```python
from build123d import *

# Parameters (mm, degrees)
F1_DEPTH = 10
F2_START = 6.1
F2_DEPTH = 3.9


with BuildPart() as f1:
    # F0 (on Front) → F1 (new body)
    with BuildSketch(Plane.XZ):
        with BuildLine():
            Line((-10.0713614853, 99.2132068528), (-89.767584656, 99.2132068528))
            Line((-89.767584656, 99.2132068528), (-204.1870618351, 99.2132068528))
            Line((-204.1870618351, 99.2132068528), (-223.9194730707, 95.7754404094))
            Line((-223.9194730707, 95.7754404094), (-214.9214308969, 56.800637818))
            Line((-214.9214308969, 56.800637818), (-199.3315098604, 60.3998546875))
            ThreePointArc((-199.3315098604, 60.3998546875), (-196.3120285861, 59.8945668129), (-194.5342253839, 57.4021786457))
            Line((-194.5342253839, 57.4021786457), (-182.4993439765, 5.2733801797))
            ThreePointArc((-182.4993439765, 5.2733801797), (-183.004631851, 2.2538989054), (-185.4970200182, 0.4760957032))
            Line((-185.4970200182, 0.4760957032), (-201.0869410548, -3.1231211663))
            Line((-201.0869410548, -3.1231211663), (-179.246252088, -97.7255385038))
            Line((-179.246252088, -97.7255385038), (-49.9194730707, -97.7255385038))
            Line((-49.9194730707, -97.7255385038), (79.4073059466, -97.7255385038))
            Line((79.4073059466, -97.7255385038), (101.2479949134, -3.1231211663))
            Line((101.2479949134, -3.1231211663), (85.6580738768, 0.4760957032))
            ThreePointArc((85.6580738768, 0.4760957032), (83.1656857096, 2.2538989054), (82.6603978351, 5.2733801797))
            Line((82.6603978351, 5.2733801797), (94.6952792425, 57.4021786457))
            ThreePointArc((94.6952792425, 57.4021786457), (96.4730824447, 59.8945668129), (99.492563719, 60.3998546875))
            Line((99.492563719, 60.3998546875), (115.0824847556, 56.800637818))
            Line((115.0824847556, 56.800637818), (124.0805269293, 95.7754404094))
            Line((124.0805269293, 95.7754404094), (104.3481156937, 99.2132068528))
            Line((104.3481156937, 99.2132068528), (-10.0713614853, 99.2132068528))
        make_face()
        with BuildLine():
            Line((-146.7194564495, -12.6849211634), (-142.1879175143, -10.5718298547))
            Line((-142.1879175143, -10.5718298547), (-69.6832945513, 23.2376310846))
            Line((-69.6832945513, 23.2376310846), (-65.1517556162, 25.3507223933))
            ThreePointArc((-65.1517556162, 25.3507223933), (-51.7296025235, 20.4654581878), (-56.614866729, 7.0433050951))
            Line((-56.614866729, 7.0433050951), (-61.1464056642, 4.9302137864))
            Line((-61.1464056642, 4.9302137864), (-133.6510286271, -28.8792471528))
            Line((-133.6510286271, -28.8792471528), (-138.1825675623, -30.9923384615))
            ThreePointArc((-138.1825675623, -30.9923384615), (-151.6047206549, -26.107074256), (-146.7194564495, -12.6849211634))
        make_face(mode=Mode.SUBTRACT)
        with BuildLine():
            Line((38.3436214209, -30.9923384615), (33.8120824857, -28.8792471528))
            Line((33.8120824857, -28.8792471528), (-38.6925404772, 4.9302137864))
            Line((-38.6925404772, 4.9302137864), (-43.2240794124, 7.0433050951))
            ThreePointArc((-43.2240794124, 7.0433050951), (-48.1093436179, 20.4654581878), (-34.6871905252, 25.3507223933))
            Line((-34.6871905252, 25.3507223933), (-30.15565159, 23.2376310846))
            Line((-30.15565159, 23.2376310846), (42.3489713729, -10.5718298547))
            Line((42.3489713729, -10.5718298547), (46.8805103081, -12.6849211634))
            ThreePointArc((46.8805103081, -12.6849211634), (51.7657745136, -26.107074256), (38.3436214209, -30.9923384615))
        make_face(mode=Mode.SUBTRACT)
        with BuildLine():
            ThreePointArc((-115.4963022827, 15.004871972), (-132.7723409168, 21.2928358008), (-126.484377088, 38.5688744349))
            Line((-126.484377088, 38.5688744349), (-117.4212992176, 42.7950570523))
            ThreePointArc((-117.4212992176, 42.7950570523), (-100.1452605835, 36.5070932235), (-106.4332244123, 19.2310545894))
            Line((-106.4332244123, 19.2310545894), (-115.4963022827, 15.004871972))
        make_face(mode=Mode.SUBTRACT)
        with BuildLine():
            Line((-90.729683986, 68.371758879), (-163.234306949, 34.5622979397))
            Line((-163.234306949, 34.5622979397), (-167.7658458841, 32.449206631))
            ThreePointArc((-167.7658458841, 32.449206631), (-181.1879989768, 37.3344708365), (-176.3027347713, 50.7566239292))
            Line((-176.3027347713, 50.7566239292), (-171.7711958361, 52.8697152379))
            Line((-171.7711958361, 52.8697152379), (-99.2665728732, 86.6791761771))
            Line((-99.2665728732, 86.6791761771), (-94.735033938, 88.7922674858))
            ThreePointArc((-94.735033938, 88.7922674858), (-81.3128808454, 83.9070032804), (-86.1981450508, 70.4848501877))
            Line((-86.1981450508, 70.4848501877), (-90.729683986, 68.371758879))
        make_face(mode=Mode.SUBTRACT)
        with BuildLine():
            ThreePointArc((26.6454309466, 38.5688744349), (32.9333947754, 21.2928358008), (15.6573561413, 15.004871972))
            Line((15.6573561413, 15.004871972), (6.594278271, 19.2310545894))
            ThreePointArc((6.594278271, 19.2310545894), (0.3063144421, 36.5070932235), (17.5823530762, 42.7950570523))
            Line((17.5823530762, 42.7950570523), (26.6454309466, 38.5688744349))
        make_face(mode=Mode.SUBTRACT)
        with BuildLine():
            Line((-0.5723732682, 86.6791761771), (71.9322496947, 52.8697152379))
            Line((71.9322496947, 52.8697152379), (76.4637886299, 50.7566239292))
            ThreePointArc((76.4637886299, 50.7566239292), (81.3490528354, 37.3344708365), (67.9268997428, 32.449206631))
            Line((67.9268997428, 32.449206631), (63.3953608076, 34.5622979397))
            Line((63.3953608076, 34.5622979397), (-9.1092621554, 68.371758879))
            Line((-9.1092621554, 68.371758879), (-13.6408010905, 70.4848501877))
            ThreePointArc((-13.6408010905, 70.4848501877), (-18.526065296, 83.9070032804), (-5.1039122034, 88.7922674858))
            Line((-5.1039122034, 88.7922674858), (-0.5723732682, 86.6791761771))
        make_face(mode=Mode.SUBTRACT)
    extrude(amount=F1_DEPTH)

    # F0 (on Front) → F2 (join)
    with BuildSketch(Plane.XZ.offset(F2_START)):
        with BuildLine():
            Line((-167.7658458841, 32.449206631), (-163.234306949, 34.5622979397))
            Line((-163.234306949, 34.5622979397), (-90.729683986, 68.371758879))
            Line((-90.729683986, 68.371758879), (-86.1981450508, 70.4848501877))
            ThreePointArc((-86.1981450508, 70.4848501877), (-81.3128808454, 83.9070032804), (-94.735033938, 88.7922674858))
            Line((-94.735033938, 88.7922674858), (-99.2665728732, 86.6791761771))
            Line((-99.2665728732, 86.6791761771), (-171.7711958361, 52.8697152379))
            Line((-171.7711958361, 52.8697152379), (-176.3027347713, 50.7566239292))
            ThreePointArc((-176.3027347713, 50.7566239292), (-181.1879989768, 37.3344708365), (-167.7658458841, 32.449206631))
        make_face()
        with BuildLine():
            Line((-155.9039639517, 42.504342484), (-164.9670418221, 38.2781598666))
            ThreePointArc((-164.9670418221, 38.2781598666), (-172.9405981148, 41.1802970184), (-170.038460963, 49.153853311))
            Line((-170.038460963, 49.153853311), (-160.9753830926, 53.3800359284))
            ThreePointArc((-160.9753830926, 53.3800359284), (-153.0018268, 50.4778987767), (-155.9039639517, 42.504342484))
        make_face(mode=Mode.SUBTRACT)
        with BuildLine():
            ThreePointArc((-97.533838, 82.9633142503), (-89.5602817074, 80.0611770985), (-92.4624188592, 72.0876208058))
            Line((-92.4624188592, 72.0876208058), (-101.5254967295, 67.8614381884))
            ThreePointArc((-101.5254967295, 67.8614381884), (-109.4990530222, 70.7635753402), (-106.5969158704, 78.7371316329))
            Line((-106.5969158704, 78.7371316329), (-97.533838, 82.9633142503))
        make_face(mode=Mode.SUBTRACT)
        with BuildLine():
            Line((76.4637886299, 50.7566239292), (71.9322496947, 52.8697152379))
            Line((71.9322496947, 52.8697152379), (-0.5723732682, 86.6791761771))
            Line((-0.5723732682, 86.6791761771), (-5.1039122034, 88.7922674858))
            ThreePointArc((-5.1039122034, 88.7922674858), (-18.526065296, 83.9070032804), (-13.6408010905, 70.4848501877))
            Line((-13.6408010905, 70.4848501877), (-9.1092621554, 68.371758879))
            Line((-9.1092621554, 68.371758879), (63.3953608076, 34.5622979397))
            Line((63.3953608076, 34.5622979397), (67.9268997428, 32.449206631))
            ThreePointArc((67.9268997428, 32.449206631), (81.3490528354, 37.3344708365), (76.4637886299, 50.7566239292))
        make_face()
        with BuildLine():
            ThreePointArc((70.1995148216, 49.153853311), (73.1016519734, 41.1802970184), (65.1280956807, 38.2781598666))
            Line((65.1280956807, 38.2781598666), (56.0650178103, 42.504342484))
            ThreePointArc((56.0650178103, 42.504342484), (53.1628806586, 50.4778987767), (61.1364369512, 53.3800359284))
            Line((61.1364369512, 53.3800359284), (70.1995148216, 49.153853311))
        make_face(mode=Mode.SUBTRACT)
        with BuildLine():
            ThreePointArc((-7.3765272822, 72.0876208058), (-10.278664434, 80.0611770985), (-2.3051081413, 82.9633142503))
            Line((-2.3051081413, 82.9633142503), (6.757969729, 78.7371316329))
            ThreePointArc((6.757969729, 78.7371316329), (9.6601068808, 70.7635753402), (1.6865505881, 67.8614381884))
            Line((1.6865505881, 67.8614381884), (-7.3765272822, 72.0876208058))
        make_face(mode=Mode.SUBTRACT)
        with BuildLine():
            Line((-69.6832945513, 23.2376310846), (-142.1879175143, -10.5718298547))
            Line((-142.1879175143, -10.5718298547), (-146.7194564495, -12.6849211634))
            ThreePointArc((-146.7194564495, -12.6849211634), (-151.6047206549, -26.107074256), (-138.1825675623, -30.9923384615))
            Line((-138.1825675623, -30.9923384615), (-133.6510286271, -28.8792471528))
            Line((-133.6510286271, -28.8792471528), (-61.1464056642, 4.9302137864))
            Line((-61.1464056642, 4.9302137864), (-56.614866729, 7.0433050951))
            ThreePointArc((-56.614866729, 7.0433050951), (-51.7296025235, 20.4654581878), (-65.1517556162, 25.3507223933))
            Line((-65.1517556162, 25.3507223933), (-69.6832945513, 23.2376310846))
        make_face()
        with BuildLine():
            ThreePointArc((-135.3837635002, -25.163385226), (-143.3573197929, -22.2612480742), (-140.4551826411, -14.2876917815))
            Line((-140.4551826411, -14.2876917815), (-131.3921047708, -10.0615091641))
            ThreePointArc((-131.3921047708, -10.0615091641), (-123.4185484781, -12.9636463159), (-126.3206856299, -20.9372026086))
            Line((-126.3206856299, -20.9372026086), (-135.3837635002, -25.163385226))
        make_face(mode=Mode.SUBTRACT)
        with BuildLine():
            Line((-62.8791405373, 8.6460757133), (-71.9422184077, 4.4198930959))
            ThreePointArc((-71.9422184077, 4.4198930959), (-79.9157747003, 7.3220302477), (-77.0136375486, 15.2955865403))
            Line((-77.0136375486, 15.2955865403), (-67.9505596782, 19.5217691577))
            ThreePointArc((-67.9505596782, 19.5217691577), (-59.9770033855, 16.6196320059), (-62.8791405373, 8.6460757133))
        make_face(mode=Mode.SUBTRACT)
        with BuildLine():
            Line((-38.6925404772, 4.9302137864), (33.8120824857, -28.8792471528))
            Line((33.8120824857, -28.8792471528), (38.3436214209, -30.9923384615))
            ThreePointArc((38.3436214209, -30.9923384615), (51.7657745136, -26.107074256), (46.8805103081, -12.6849211634))
            Line((46.8805103081, -12.6849211634), (42.3489713729, -10.5718298547))
            Line((42.3489713729, -10.5718298547), (-30.15565159, 23.2376310846))
            Line((-30.15565159, 23.2376310846), (-34.6871905252, 25.3507223933))
            ThreePointArc((-34.6871905252, 25.3507223933), (-48.1093436179, 20.4654581878), (-43.2240794124, 7.0433050951))
            Line((-43.2240794124, 7.0433050951), (-38.6925404772, 4.9302137864))
        make_face()
        with BuildLine():
            ThreePointArc((40.6162364998, -14.2876917815), (43.5183736515, -22.2612480742), (35.5448173589, -25.163385226))
            Line((35.5448173589, -25.163385226), (26.4817394885, -20.9372026086))
            ThreePointArc((26.4817394885, -20.9372026086), (23.5796023367, -12.9636463159), (31.5531586294, -10.0615091641))
            Line((31.5531586294, -10.0615091641), (40.6162364998, -14.2876917815))
        make_face(mode=Mode.SUBTRACT)
        with BuildLine():
            ThreePointArc((-36.9598056041, 8.6460757133), (-39.8619427558, 16.6196320059), (-31.8883864632, 19.5217691577))
            Line((-31.8883864632, 19.5217691577), (-22.8253085928, 15.2955865403))
            ThreePointArc((-22.8253085928, 15.2955865403), (-19.923171441, 7.3220302477), (-27.8967277337, 4.4198930959))
            Line((-27.8967277337, 4.4198930959), (-36.9598056041, 8.6460757133))
        make_face(mode=Mode.SUBTRACT)
    extrude(amount=F2_DEPTH)


solid = f1.part
```
Can you work these out from the model? Positions are in its coordinate system, mm. A direction names the side the tool comes from. Coordinates: 2 decimals unless noted, no trailing zeros. Loops run counter-clockwise (first coordinate to the right, second up) from the corner with the lowest first, then second, coordinate; pieces in that order, holes last.
Item 1: Suppose I cut it at B-B (z = -42.5). Please give me the cut outline in (x, y).
Answers below:
outline: (-192, -10) - (92.16, -10) - (92.16, 0) - (-192, 0) - close
Item 2: I'm going to push flat-ended pins straight in: pin 1 (1 mm diameter, centred on y = -3, z = 38.5, fed in from -X); pin 2 (3 mm diameter, centred on y = -7.5, z = 77.5, fed in from -X); pin 3 (4 mm diameter, centred on y = -7.5, z = 49, fed in from +X). Where does each tip first touch, or does it pass through?
Answers below:
pin 1: stops at x = -190.29
pin 2: stops at x = -220.05
pin 3: stops at x = 93.22
Item 3: Which directions (+Z, -Z, +X, -X, +Y, -Y) give clear straight access to the entire face, cutting with the end or side of a thin tool? Please do faces 4 (the face through (-110.9, -4.93, 17.15)), 5 (the face through (-102, -6.1, -5)), 6 (the face through (-193.183, -4.93, -1.298)).
Answers below:
face 4: +Y, -Y
face 5: +Y
face 6: -X, +Y, -Y
Item 4: Suppose I cut it at A-A (y = -4.5). State how many separate pieces and enclosed holes the cut face has, then the cut area to 3 significant figures.
Answers below:
separate pieces: 1
enclosed holes: 6
area: 47,200 mm2
Item 5: If we mould it in two halves opening along Z, with no side actions, what happens to faces 1 (the face through (90.175, -4.93, -51.087)), 2 (the face through (-48, -5, 99.213)), 3 (the face through (-89.617, -8.023, 80.18))? For each: released by +Z, released by -Z, zero draft, split by the parting line, or undercut.
Answers below:
face 1: released by -Z
face 2: released by +Z
face 3: undercut
Item 6: Please list where these lines run through material, in increasing order: L1, parallel to Z at x = -106.5, y = -9.5; L2, parallel to Z at x = 21, y = -4.75; L3, parallel to X at y = -5.75, z = 16.
Answers below:
L1: z = -97.73 to 19.2, 42.83 to 67.82, 78.78 to 99.21
L2: z = -97.73 to -22.9, -0.62 to 13.79, 41.2 to 54.33, 76.62 to 99.21
L3: x = -184.98 to -128.25, -113.36 to -85.2, -50.79 to -49.05, -14.63 to 13.52, 28.41 to 85.14
